Design review of the part built by this model. Coordinates are the model's own, in mm. Face numbers are marked on the shaded views. A direction names the side the tool comes from. Give positions to 0.01 mm unless a question says otherwise; leave off trailing zeros. Write each loop counter-clockwise with the first axis right and the second up, starting at its lowest first coordinate (ties: lowest second). Pieces come first, ordered by that corner, then holes. Notation, with made-up numbers: M 6.5,7 L 46.5,7 A22 ccw 46.5,33 Z; hole C 81.5,55 d11. An arc over 180 degrees is marked long. Use a Markdown table: item, result. Add a question column.
```python
from build123d import *

# Parameters (mm, degrees)
EXTRUDE_1_DEPTH = 30
EXTRUDE_2_DEPTH = 70


with BuildPart() as part:
    # 草图1 → 凸台-拉伸1 (new body)
    with BuildSketch(Plane(origin=(0, 0, 0), x_dir=(1, 0, 0), z_dir=(0, 1, 0))):
        with BuildLine():
            Line((75.055476805, 35), (35.707142143, 35))
            ThreePointArc((35.707142143, 35), (46.289075964, 18.902948088), (50, 0))
            ThreePointArc((50, 0), (46.289075964, -18.902948088), (35.707142143, -35))
            Line((35.707142143, -35), (75.055476805, -35))
            Line((75.055476805, -35), (75.055476805, 35))
        make_face()
        with BuildLine():
            Line((0.055476805, -35), (0.055476805, 35))
            Line((0.055476805, 35), (35.707142143, 35))
            ThreePointArc((35.707142143, 35), (-50, 0), (35.707142143, -35))
            Line((35.707142143, -35), (0.055476805, -35))
        make_face()
        with BuildLine():
            Line((35.707142143, 35), (0.055476805, 35))
            Line((0.055476805, 35), (0.055476805, -35))
            Line((0.055476805, -35), (35.707142143, -35))
            ThreePointArc((35.707142143, -35), (46.289075964, -18.902948088), (50, 0))
            ThreePointArc((50, 0), (46.289075964, 18.902948088), (35.707142143, 35))
        make_face()
    extrude(amount=EXTRUDE_1_DEPTH)

    # 草图2 → 凸台-拉伸2 (add)
    with BuildSketch(Plane.XY.offset(35)):
        Polygon((75.055476805, 0), (140.174133177, 114.192122372), (140.174133177, 191.411564081), (120.26890055, 191.411564081), (120.26890055, 109.286292207), (75.055476805, 30), align=None)
    extrude(amount=-EXTRUDE_2_DEPTH)


solid = part.part
```
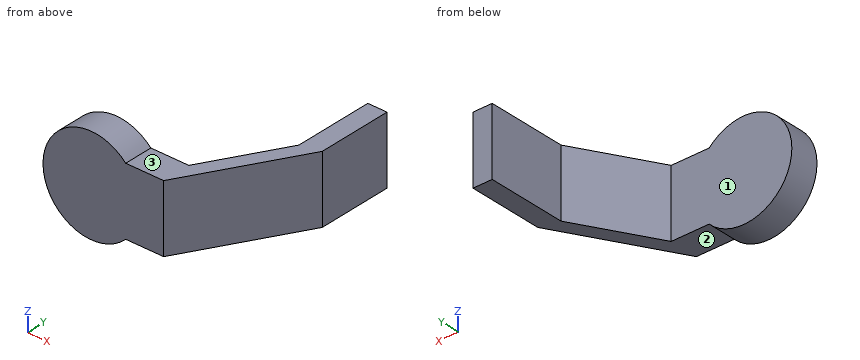
(1) Machinability: for the marked faces 1, 2 and 3, which of the approach directions +Z, -Z, +X, -X, +Y, -Y give a long, thin tool a straight path to every point of the face, cutting with its end or side? Answer none if there is none.
(2) Add section A-A on z = 0. Give the boundary of the cut face in (x, y), then the cut area to 3 significant figures.
(3) For pin 1 (1.5 mm diameter, centred on x = -10, z = 34, fed in from +Y); pin 2 (8 mm diameter, centred on x = 42.5, z = 32.5, fed in from -Y); pin 3 (10 mm diameter, centred on x = 112.5, z = -11.5, fed in from +Y); pin 4 (6 mm diameter, centred on y = 24.5, z = 6, fed in from -X), all flat-tipped, find the tip position at first contact; note any pin that passes through.
(4) Add section C-C on y = 169. Give the boundary of the cut face in (x, z).
(5) Wall thickness on L1, parallel to Y at x = -6, z = -17.5; L2, parallel to Z at x = 132, y = 112; L3, parallel to X at y = 82, z = -22: over which ranges is each line inside the solid? List them lowest first.
(6) Add section B-B on x = 53.5. Give the boundary of the cut face in (y, z), then the cut area to 3 significant figures.
(7) Add section D-D on z = -31. Give the boundary of the cut face in (x, y), then the cut area to 3 significant figures.
From the geometry:
| question | item | result |
|---|---|---|
| 1 | face 1 | +Z, -Z, -X, +Y |
| 1 | face 2 | -Z, +X, +Y, -Y |
| 1 | face 3 | +Z, +X, +Y, -Y |
| 2 | outline | M -50,0 L 75.06,0 L 140.17,114.19 L 140.17,191.41 L 120.27,191.41 L 120.27,109.29 L 75.06,30 L -50,30 Z |
| 2 | area | 6,990 mm^2 |
| 3 | pin 1 | stops at y = 30 |
| 3 | pin 2 | stops at y = 0 |
| 3 | pin 3 | stops at y = 104.43 |
| 3 | pin 4 | stops at x = -49.91 |
| 4 | outline | M 120.27,-35 L 140.17,-35 L 140.17,35 L 120.27,35 Z |
| 5 | L1 | y = 0 to 30 |
| 5 | L2 | z = -35 to 35 |
| 5 | L3 | x = 104.71 to 121.82 |
| 6 | outline | M 0,-35 L 30,-35 L 30,35 L 0,35 Z |
| 6 | area | 2,100 mm^2 |
| 7 | outline | M -39.23,0 L 75.06,0 L 140.17,114.19 L 140.17,191.41 L 120.27,191.41 L 120.27,109.29 L 75.06,30 L -39.23,30 Z |
| 7 | area | 6,670 mm^2 |
